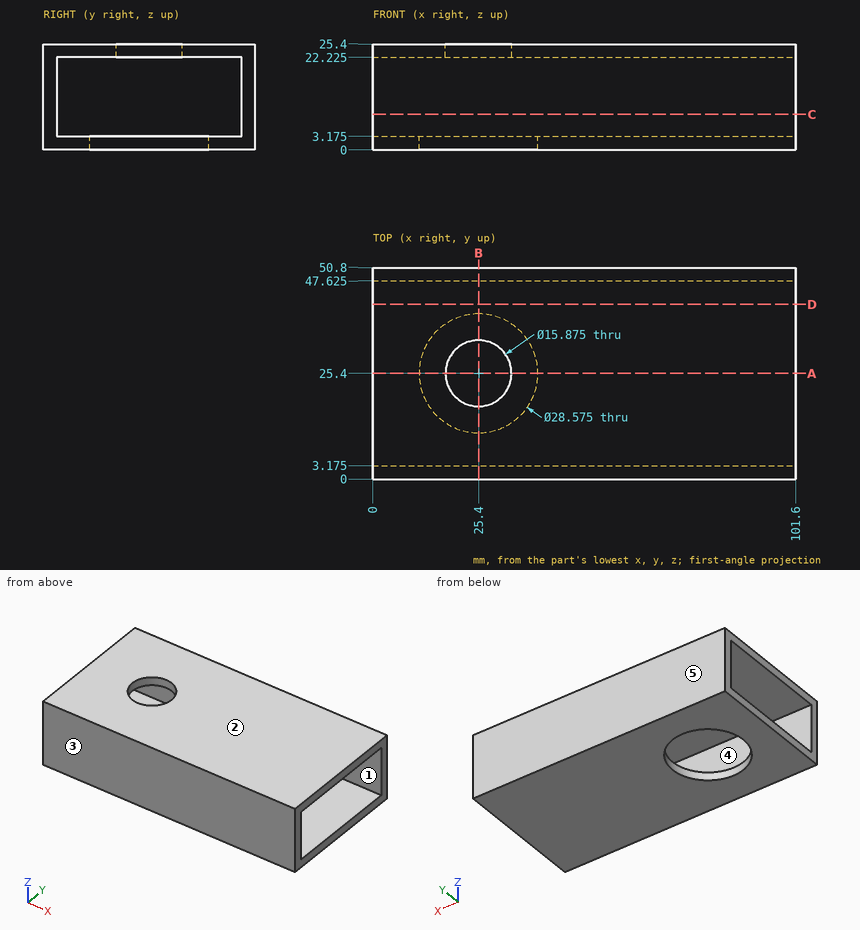
Design review of the part shown in the three views and the two pictorial views. Dimensions are in mm from the part's minimum x, y and z. A direction names the side the tool comes from. Coordinates: 2 decimals unless noted, no trailing zeros. Order: outer loops, then holes, each group sorted by start corner. A loop starts at its lowest first (then second) coordinate and runs counter-clockwise, first axis right, second up. Notation, with made-up numbers: (-19.5, -17.5) - (-15.5, -17.5) arc R10 cw to (-15.5, 0.5) - close; hole circle Ø2 at (33, 57.5). An arc over 180 degrees is marked (long way). One line per question, with ' | ' between items.
Q1. Clearance check with a flat-ended pin moving along its axis: pin 1 Ø5.5 at (x, z) = (40.5, 14) entering from -Y. State where the tip first meets the part, or that it passes through.
Answer key:
pin 1: stops at y = 0
Q2. To check wall thickness, follow line 1 along Z through (x, y) = (67, 9.5) (3 decimals); line 2 along X through (y, z) = (25.4, 23.45); line 3 along Y through (x, z) = (17.5, 21.75) (3 decimals). State the ranges of each line that lie inside material, in increasing order.
Answer key:
line 1: z = 0 to 3.175, 22.225 to 25.4 | line 2: x = 0 to 17.46, 33.34 to 101.6 | line 3: y = 0 to 3.175, 47.625 to 50.8
Q3. For the marked faces 4 and 5, list the 3-axis set-ups (+Z, -Z, +X, -X, +Y, -Y) from which the entire face can be reached by the end or side of a thin tool; tool diameter is ignored.
Answer key:
face 4: +X, -X | face 5: +Z, -Z, +X, -X, +Y
Q4. Consider section B-B, the plane x = 25.4. Give the boundary of the cut face in (y, z) (1 decimal).
Answer key:
outline: (0, 0) - (11.1, 0) - (11.1, 3.2) - (3.2, 3.2) - (3.2, 22.2) - (17.5, 22.2) - (17.5, 25.4) - (0, 25.4) - close; (33.3, 22.2) - (47.6, 22.2) - (47.6, 3.2) - (39.7, 3.2) - (39.7, 0) - (50.8, 0) - (50.8, 25.4) - (33.3, 25.4) - close
Q5. Consider section C-C, the plane z = 8.5. Give the boundary of the cut face in (x, y) (3 decimals), then the cut area to 3 significant figures.
Answer key:
outline: (0, 0) - (101.6, 0) - (101.6, 3.175) - (0, 3.175) - close; (0, 47.625) - (101.6, 47.625) - (101.6, 50.8) - (0, 50.8) - close | area: 645 mm2
Q6. Consider section D-D, the plane y = 42. Give the boundary of the cut face in (x, z) (3 decimals).
Answer key:
outline: (0, 0) - (101.6, 0) - (101.6, 3.175) - (0, 3.175) - close; (0, 22.225) - (101.6, 22.225) - (101.6, 25.4) - (0, 25.4) - close
Q7. Consider section A-A, the plane y = 25.4. Give the boundary of the cut face in (x, z) (1 decimal), then the cut area to 3 significant figures.
Answer key:
outline: (0, 0) - (11.1, 0) - (11.1, 3.2) - (0, 3.2) - close; (0, 22.2) - (17.5, 22.2) - (17.5, 25.4) - (0, 25.4) - close; (33.3, 22.2) - (101.6, 22.2) - (101.6, 25.4) - (33.3, 25.4) - close; (39.7, 0) - (101.6, 0) - (101.6, 3.2) - (39.7, 3.2) - close | area: 504 mm2
Q8. The part is to be moulded in two halves that separate along Z. For the marked faces 1, 2 and 3, say which applies: +Z half, -Z half, draft (parallel to the pull), parting line (faces both ways), or undercut.
Answer key:
face 1: undercut | face 2: +Z half | face 3: draft
